Answer from the drawing. Dimensions are ordinates in mm from the lowest x, y and z of the part. Give positions to 0.01 mm unless a question says otherwise; leave off trailing zeros. Write each loop counter-clockwise with the first axis right and the second up, starting at its lowest first coordinate (ties: lowest second). Pieces come first, ordered by that corner, then holes.
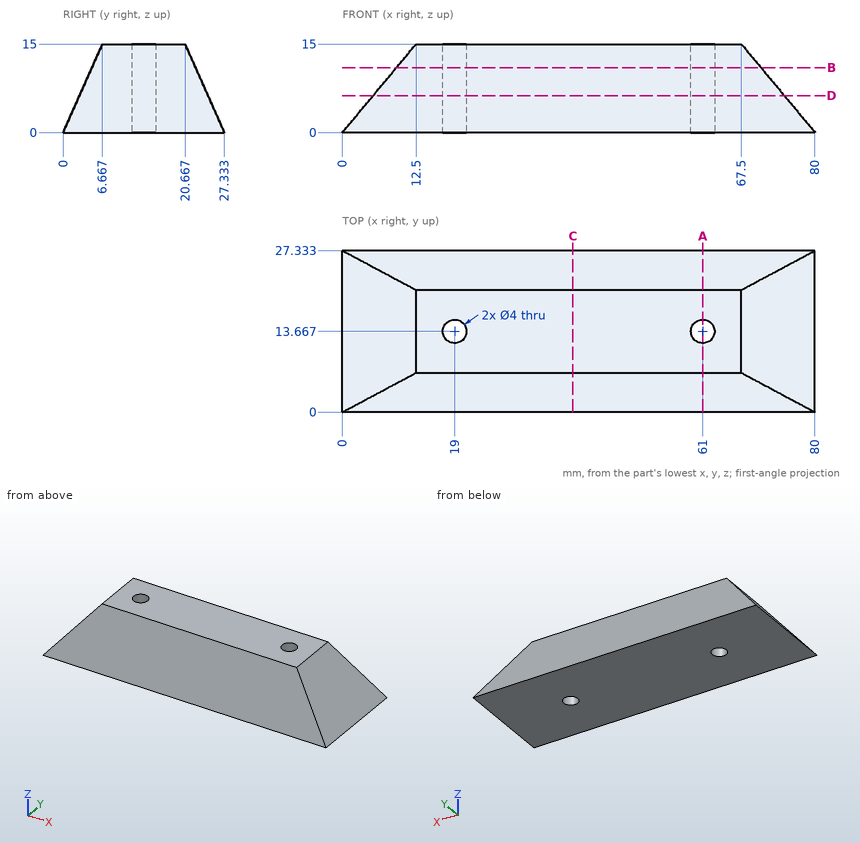
Item 1: Section D-D (z = 6.25) is taken. Write down the section's boundary in (x, y) (1 decimal).
Result set:
outline: (5.2, 2.8) - (74.8, 2.8) - (74.8, 24.6) - (5.2, 24.6) - close; hole circle Ø4 at (19, 13.7); hole circle Ø4 at (61, 13.7)
Item 2: Section A-A (x = 61) is taken. Write down the section's boundary in (y, z), and give its area (3 significant figures).
Result set:
outline: (0, 0) - (11.67, 0) - (11.67, 15) - (6.67, 15) - close; (15.67, 0) - (27.33, 0) - (20.67, 15) - (15.67, 15) - close
area: 250 mm2
Item 3: Section B-B (z = 11) is taken. Write down the section's boundary in (x, y) (1 decimal).
Result set:
outline: (9.2, 4.9) - (70.8, 4.9) - (70.8, 22.4) - (9.2, 22.4) - close; hole circle Ø4 at (19, 13.7); hole circle Ø4 at (61, 13.7)
Item 4: Each of these flat-tipped pins is pushed along its axis until it touches: pin 1 Ø6 at (x, z) = (59.5, 5) entering from +Y (1 decimal); pin 2 Ø3.5 at (x, y) = (61, 13.67) entering from -Z; pin 3 Ø1.5 at (y, z) = (15.5, 4.5) entering from -X (1 decimal); pin 4 Ø8 at (x, z) = (59.5, 9) entering from -Y. Where does it stop, or does it pass through?
Result set:
pin 1: stops at y = 26.4
pin 2: passes through
pin 3: stops at x = 3.1
pin 4: stops at y = 2.22
Item 5: Section C-C (x = 39) is taken. Write down the section's boundary in (y, z).
Result set:
outline: (0, 0) - (27.33, 0) - (20.67, 15) - (6.67, 15) - close
Item 6: Find the intervals of material crossed by line 1 along X through (y, z) = (14, 12); line 2 along X through (y, z) = (15.25, 8.5) (1 decimal); line 3 along Y through (x, z) = (61, 7.75) (1 decimal), in increasing order.
Result set:
line 1: x = 10 to 17.03, 20.97 to 59.03, 62.97 to 70
line 2: x = 7.1 to 17.8, 20.2 to 59.8, 62.2 to 72.9
line 3: y = 3.4 to 11.7, 15.7 to 23.9
